Input: part model. Units: mm. Frame: model coordinates. Round coordinates to 2 decimals unless told otherwise and drop trailing zeros. Write each loop counter-clockwise with the first axis right and the second up, starting at its lowest first coordinate (ties: lowest second). Pieces come first, ordered by that corner, then holes. Notation, with made-up numbers: M 65.5,77.5 L 104.5,77.5 A13 cw 104.5,87.5 Z; hole C 40,16 d11. An arc over 180 degrees is marked long. Write each question's results on one line, items separated by ' | '. Start each with the question number.
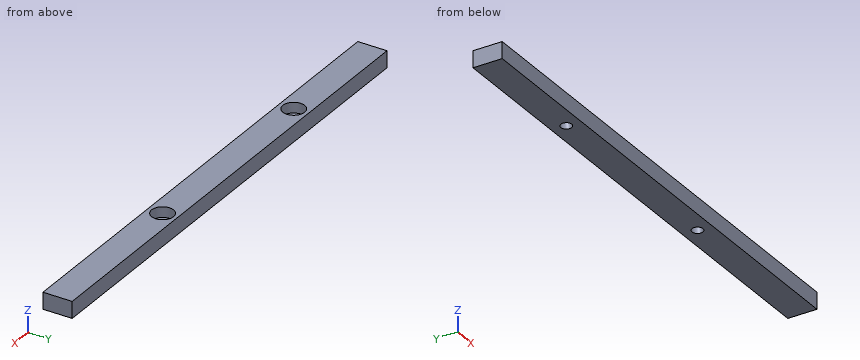
```python
from build123d import *

# Parameters (mm, degrees)
F0_W     = 240
F0_H     = 14
F1_DEPTH = 8
F2_R     = 2.6
F3_DEPTH = 8.001
F2_R_2   = 5.25
F4_DEPTH = 5


with BuildPart() as f1:
    # F0 (on Top) → F1 (new body)
    with BuildSketch(Plane.XY):
        Rectangle(F0_W, F0_H)
    extrude(amount=F1_DEPTH)

    # F2 (on face) → F3 (cut, through all)
    with BuildSketch(Plane.XY.offset(8)):
        with Locations((-60, 0)):
            Circle(F2_R)
        with Locations((40, 0)):
            Circle(F2_R)
    extrude(amount=-F3_DEPTH, mode=Mode.SUBTRACT)

    # F2 (on face) → F4 (cut)
    with BuildSketch(Plane.XY.offset(8)):
        with Locations((-60, 0)):
            Circle(F2_R_2)
        with Locations((-60, 0)):
            Circle(F2_R, mode=Mode.SUBTRACT)
        with Locations((40, 0)):
            Circle(F2_R_2)
        with Locations((40, 0)):
            Circle(F2_R, mode=Mode.SUBTRACT)
    extrude(amount=-F4_DEPTH, mode=Mode.SUBTRACT)


solid = f1.part
```
1. Contact query for a flat-ended pin moving along its axis: P1, Ø3, axis at x = -60.5, y = 0, coming from the +Z side. Output: stop coordinate, or through.
2. Cut plane A-A on x = -60. Output: boundary loops of the cut face in (y, z), and give its area (3 significant figures).
3. Cut plane B-B on y = 0. Output: boundary loops of the cut face in (x, z), and give its area (3 significant figures).
4. Cut plane C-C on z = 5.75. Output: boundary loops of the cut face in (x, y), and give its area (3 significant figures).
5. Line query: L1, parallel to X at y = 0.5, z = 2.25; L2, parallel to X at y = 3.5, z = 4.5; L3, parallel to Y at x = -60, z = 1.25. Output: solid intervals per line, ascending. Write a range as from..to.
Answers follow:
1) P1: passes through
2) outline: M -7,0 L -2.6,0 L -2.6,3 L -5.25,3 L -5.25,8 L -7,8 Z; M 2.6,0 L 7,0 L 7,8 L 5.25,8 L 5.25,3 L 2.6,3 Z | area: 43.9 mm2
3) outline: M -120,0 L -62.6,0 L -62.6,3 L -65.25,3 L -65.25,8 L -120,8 Z; M -57.4,0 L 37.4,0 L 37.4,3 L 34.75,3 L 34.75,8 L -54.75,8 L -54.75,3 L -57.4,3 Z; M 42.6,0 L 120,0 L 120,8 L 45.25,8 L 45.25,3 L 42.6,3 Z | area: 1,780 mm2
4) outline: M -120,-7 L 120,-7 L 120,7 L -120,7 Z; hole C -60,0 d10.5; hole C 40,0 d10.5 | area: 3,190 mm2
5) L1: x = -120..-62.55, -57.45..37.45, 42.55..120 | L2: x = -120..-63.91, -56.09..36.09, 43.91..120 | L3: y = -7..-2.6, 2.6..7
